Could you check a few things on this model? Use its own coordinates, in mm. A direction names the side the tool comes from. Give positions to 0.01 mm unless a question says otherwise; leave off trailing zeros. Write each question's results on one line, items separated by ' | '. Start each with the question number.
1) If we mould it in two halves opening along Z, with no side actions, what happens to faces 4 (the face through (3.6, 23.16, -36.76)), 5 (the face through (2, -44.025, 0)), 6 (the face through (3.6, -43.42, -1.68)), 7 (the face through (2.07, 21.99, 38.14))? For each: +Z half, -Z half, draft (parallel to the pull), parting line (faces both ways), or undercut.
2) On a 3-axis mill with a long thin cutter (end or side, diameter ignored), from which of +Z, -Z, +X, -X, +Y, -Y can I reach the whole of each face in a straight line? I mean faces 1 (the face through (-2.6, 37.2, -15.4)), 2 (the face through (2, -2, 42.9)), 3 (the face through (2.07, 21.44, -37.07)). Say none if no direction works.
3) I'm going to push flat-ended pins straight in: pin 1 (4 mm diameter, centred on x = -2, y = 33.5, fed in from -Z); pin 2 (0.6 mm diameter, centred on y = -36.5, z = 24, fed in from -X); pin 3 (6 mm diameter, centred on x = -2, z = -20, fed in from -Y). Where does each tip first touch, or does it pass through?
4) If I drill on probe 1 along Z at (x, y) = (-1.2, 0); probe 2 along Z at (x, y) = (-3.4, 0), over which ranges is the centre line in solid material (lowest first)? Write a range as [from, to].
from build123d import *

# Parameters (mm, degrees)
BOX003_W        = 2
BOX003_H        = 3
BOX003_DEPTH    = 10
ARRAY004_COUNT  = 6
BOX004_W        = 2
BOX004_H        = 3
BOX004_DEPTH    = 10
ARRAY003_COUNT  = 6
BOX001_W        = 5
BOX001_H        = 1.2
BOX001_DEPTH    = 10
ARRAY002_COUNT  = 6
CHAMFER_SIZE    = 2
CHAMFER001_SIZE = 2
BOX002_W        = 4.2
BOX002_H        = 1.2
BOX002_DEPTH    = 4.5
ARRAY_COUNT     = 3
BOX_W           = 4.4
BOX_H           = 5.25
BOX_DEPTH       = 1.2
ARRAY001_COUNT  = 6
CHAMFER002_SIZE = 1
FILLET_R        = 2


with BuildPart() as array004:
    # Box003 → Box003 (new body)
    with BuildSketch(Plane(origin=(0, -5.5, 38), x_dir=(1, 0, 0), z_dir=(0, 0, 1))):
        with Locations((1, 1.5)):
            Rectangle(BOX003_W, BOX003_H)
    extrude(amount=BOX003_DEPTH)

    # Array004: Array004 ×6 about axis
    array004_axis = Axis((0, 0, 0), (1, 0, 0))


with BuildPart() as array004_1:
    add(array004.part)
    for i in range(1, ARRAY004_COUNT):
        add(array004.part.rotate(array004_axis, i * 360 / ARRAY004_COUNT))


with BuildPart() as array003:
    # Box004 → Box004 (new body)
    with BuildSketch(Plane(origin=(0, 2.5, 38), x_dir=(1, 0, 0), z_dir=(0, 0, 1))):
        with Locations((1, 1.5)):
            Rectangle(BOX004_W, BOX004_H)
    extrude(amount=BOX004_DEPTH)

    # Array003: Array003 ×6 about axis
    array003_axis = Axis((0, 0, 0), (1, 0, 0))


with BuildPart() as array003_1:
    add(array003.part)
    for i in range(1, ARRAY003_COUNT):
        add(array003.part.rotate(array003_axis, i * 360 / ARRAY003_COUNT))


with BuildPart() as array002:
    # Box001 → Box001 (new body)
    with BuildSketch(Plane(origin=(0, -0.6, 38), x_dir=(1, 0, 0), z_dir=(0, 0, 1))):
        with Locations((2.5, 0.6)):
            Rectangle(BOX001_W, BOX001_H)
    extrude(amount=BOX001_DEPTH)

    # Array002: Array002 ×6 about axis
    array002_axis = Axis((0, 0, 0), (1, 0, 0))


with BuildPart() as array002_1:
    add(array002.part)
    for i in range(1, ARRAY002_COUNT):
        add(array002.part.rotate(array002_axis, i * 360 / ARRAY002_COUNT))


with BuildPart() as chamfer001:
    # Sketch → Revolution (revolve)
    with BuildSketch(Plane.XY):
        Polygon((-6, 44.4), (0, 44.4), (0, 42.1), (-2.6, 42.1), (-2.6, 40.1), (-6, 40.1), align=None)
    revolve(axis=Axis((0, 0, 0), (1, 0, 0)))

    # Chamfer
    chamfer_edges = [chamfer001.edges().sort_by_distance(p)[0] for p in [
        (-6, -44.4, 0),
    ]]
    chamfer(chamfer_edges, length=CHAMFER_SIZE)

    # Chamfer001
    chamfer001_edges = [chamfer001.edges().sort_by_distance(p)[0] for p in [
        (-6, -40.1, 0),
    ]]
    chamfer(chamfer001_edges, length=CHAMFER001_SIZE)


with BuildPart() as fusion:
    # Box002 → Box002 (new body)
    with BuildSketch(Plane(origin=(0, -44.025, -2.25), x_dir=(1, 0, 0), z_dir=(0, 0, 1))):
        with Locations((2.1, 0.6)):
            Rectangle(BOX002_W, BOX002_H)
    extrude(amount=BOX002_DEPTH)

    # Array: Fusion ×3 about axis
    array_axis = Axis((0, 0, 0), (1, 0, 0))


with BuildPart() as fusion_1:
    add(fusion.part)
    for i in range(1, ARRAY_COUNT):
        add(fusion.part.rotate(array_axis, i * 360 / ARRAY_COUNT))

    # Fusion: union Chamfer001
    add(chamfer001.part)


with BuildPart() as fillet_body:
    # Box → Box (new body)
    with BuildSketch(Plane(origin=(0, -2.625, 42.9), x_dir=(1, 0, 0), z_dir=(0, 0, 1))):
        with Locations((2.2, 2.625)):
            Rectangle(BOX_W, BOX_H)
    extrude(amount=BOX_DEPTH)

    # Array001: Fillet body ×6 about axis
    array001_axis = Axis((0, 0, 0), (1, 0, 0))


with BuildPart() as fillet_body_1:
    add(fillet_body.part)
    for i in range(1, ARRAY001_COUNT):
        add(fillet_body.part.rotate(array001_axis, i * 360 / ARRAY001_COUNT))

    # Fusion001: union Fusion
    add(fusion_1.part)

    # Cut: cut Array002
    add(array002_1.part, mode=Mode.SUBTRACT)

    # Cut001: cut Array003
    add(array003_1.part, mode=Mode.SUBTRACT)

    # Cut002: cut Array004
    add(array004_1.part, mode=Mode.SUBTRACT)

    # Chamfer002
    chamfer002_edges = [fillet_body_1.edges().sort_by_distance(p)[0] for p in [
        (4.4, -38.984605, 19.476683),
        (4.4, -38.984605, -19.476683),
        (4.4, 38.984605, -19.476683),
        (4.4, 36.359605, 24.023317),
        (4.4, 36.359605, -24.023317),
        (4.4, -36.359605, -24.023317),
        (4.4, 38.984605, 19.476683),
        (4.4, -36.359605, 24.023317),
        (4.4, 2.625, -43.5),
        (4.4, -2.625, -43.5),
        (4.4, 2.625, 43.5),
        (4.4, -2.625, 43.5),
    ]]
    chamfer(chamfer002_edges, length=CHAMFER002_SIZE)

    # Fillet
    fillet_edges = [fillet_body_1.edges().sort_by_distance(p)[0] for p in [
        (4.2, 23.661057, 36.482153),
        (4.2, 19.763943, 38.732153),
        (4.2, 19.763943, -38.732153),
        (4.2, 23.661057, -36.482153),
        (4.2, -43.425, 2.25),
        (4.2, -43.425, -2.25),
    ]]
    fillet(fillet_edges, radius=FILLET_R)


solid = fillet_body_1.part
Answers:
1) face 4: undercut | face 5: draft | face 6: -Z half | face 7: +Z half
2) face 1: +X | face 2: +X, +Y, -Y | face 3: +X, -Y
3) pin 1: stops at z = -31.29 | pin 2: stops at x = -5.02 | pin 3: stops at y = -41.02
4) probe 1: z = [-44.4, -42.1], [42.1, 44.4] | probe 2: z = [-44.4, -40.1], [40.1, 44.4]
